Could you check a few things on this drawing? It's one solid part, dimensions in mm from its lowest x, y, z. Coordinates: 2 decimals unless noted, no trailing zeros. Loops run counter-clockwise (first coordinate to the right, second up) from the corner with the lowest first, then second, coordinate; pieces in that order, holes last. Notation, with made-up numbers: (24.25, -7) -> (51.25, -7) arc R25 cw to (51.25, 26) -> close; hole circle Ø11 at (16.5, 28). An arc over 180 degrees is marked (long way). One line per question, with ' | ' between items.
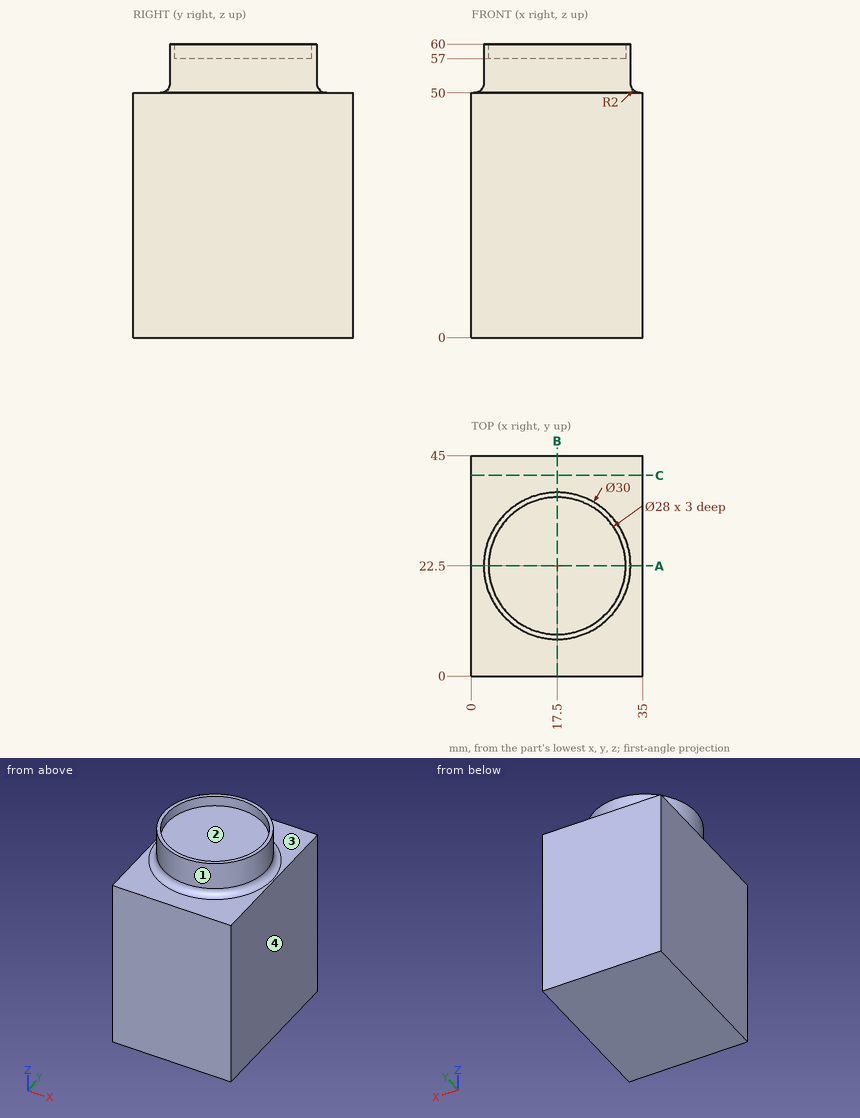
1) If we section it at A-A on y = 22.5: Please give me the cut outline in (x, z).
Data:
outline: (0, 0) -> (35, 0) -> (35, 50) -> (34.5, 50) arc R2 cw to (32.5, 52) -> (32.5, 60) -> (31.5, 60) -> (31.5, 57) -> (3.5, 57) -> (3.5, 60) -> (2.5, 60) -> (2.5, 52) arc R2 cw to (0.5, 50) -> (0, 50) -> close
2) We'd pull the mould along X, two halves only. Please class the marked faces 1, 2, 3 and 4: pulls with the +X half, pulls with the -X half, needs draft (parallel to the pull), parting line crosses it, or undercut.
Data:
face 1: parting line crosses it | face 2: undercut | face 3: needs draft | face 4: pulls with the +X half
3) I need wall thicknesses on line 1 along Y through (x, z) = (17, 58); line 2 along X through (y, z) = (22, 58); line 3 along Z through (x, y) = (26, 42). Which ranges of each line are inside material? Lowest first, please. Write a range as from..to.
Data:
line 1: 7.51..8.51, 36.49..37.49 | line 2: 2.51..3.51, 31.49..32.49 | line 3: 0..50
4) If we section it at B-B on x = 17.5: Please give me the cut outline in (y, z).
Data:
outline: (0, 0) -> (45, 0) -> (45, 50) -> (39.5, 50) arc R2 cw to (37.5, 52) -> (37.5, 60) -> (36.5, 60) -> (36.5, 57) -> (8.5, 57) -> (8.5, 60) -> (7.5, 60) -> (7.5, 52) arc R2 cw to (5.5, 50) -> (0, 50) -> close
5) I'm going to push a flat-ended pin straight in: pin 1 Ø1 at (x, z) = (26.5, 52.5) entering from +Y. Where does the tip first touch, or does it pass through?
Data:
pin 1: y = 34.86
6) If we section it at C-C on y = 41: Please give me the cut outline in (x, z).
Data:
outline: (0, 0) -> (35, 0) -> (35, 50) -> (0, 50) -> close
